Autodesk Inventor part; units mm, degrees
ref_plane "Work Plane6" through (0, -38.4796, -26.2038) normal (0, 0, -1) x (-1, 0, 0)
ref_plane "Work Plane3" through (0, 0, 0) normal (-1, 0, 0) x (0, 0, 1)
ref_plane "Work Plane1" through (0, -38.4796, -36.2038) normal (0, 0, -1) x (-1, 0, 0)
sketch "Sketch1" plane through (0, 0, 0) normal (1, 0, 0) x (0, 1, 0)
  circle A0 centre (-12.8712, -19.8017) radius 2.1703
  circle A1 centre (-32.0775, -0.5955) radius 2.1703
  circle A2 centre (31.9433, -0.5955) radius 2.1703
  circle A3 centre (31.9433, 13.4891) radius 2.1703
  circle A4 centre (-32.0775, 13.4891) radius 2.1703
  circle A5 centre (12.7371, -19.8017) radius 2.1703
  line L0 (38.3454, 26.2933) -> (38.3454, -26.2038)
  line L1 (-38.4796, 26.2933) -> (38.3454, 26.2933)
  line L2 (-38.4796, 26.2933) -> (-38.4796, -26.2038)
  line L3 (38.3454, -26.2038) -> (-38.4796, -26.2038)
  circle A6 centre (-32.0775, 13.4891) radius 2.1703
  circle A7 centre (-32.0775, -0.5955) radius 2.1703
  line L4 (11.5, -7) -> (-11.5, -7)
  line L5 (-11.5, -7) -> (-11.5, 7)
  line L6 (-11.5, 7) -> (11.5, 7)
  line L7 (11.5, 7) -> (11.5, -7)
  line L8 (11.5, -7) -> (-11.5, 7) construction
  line L9 (-11.5, -7) -> (11.5, 7) construction
  circle A8 centre (13.2, 0) radius 1
  circle A9 centre (-14, 0) radius 1
  point P0 (0, 0)
  point P1 (-11.5, 0)
  dimension "d26" = 23
  dimension "d27" = 14
  dimension "d28" = 27.2
  dimension "d29" = 2
  dimension "d30" = 2.5
ref_plane "Work Plane6" through (0, -38.4796, -26.2038) normal (0, 0, -1) x (-1, 0, 0)
sketch "Sketch3" plane through (0, -38.4796, -26.2038) normal (0, 0, -1) x (-1, 0, 0)
  line L0 (0, 76.825) -> (-3, 76.825)
  line L1 (0, 0) -> (-3, 0)
  line L2 (-3, 76.825) -> (0, 76.825)
  line L3 (0, 76.825) -> (0, 0)
  line L4 (0, 0) -> (-3, 0)
  line L5 (-3, 0) -> (-3, 76.825)
  line L6 (0, 0) -> (0, 76.825)
  line L7 (-3, 0) -> (-3, 76.825)
  line L8 (0.01, -0.01) -> (0.01, 76.835)
  line L9 (0.01, 76.835) -> (-3.01, 76.835)
  line L10 (-3.01, 76.835) -> (-3.01, -0.01)
  line L11 (-3.01, -0.01) -> (0.01, -0.01)
  point P0 (0, 38.4796)
  dimension "d3" = 0.01
extrude "Extrusion2" add sketch "Sketch3" along normal blind 10 contours L3 L1 L5 L0
ref_plane "Work Plane3" through (0, 0, 0) normal (-1, 0, 0) x (0, 0, 1)
sketch "Sketch4" plane through (0, 0, 0) normal (-1, 0, 0) x (0, 0, 1)
  line L0 (26.2933, -38.4796) -> (-36.2038, -38.4796)
  line L1 (-36.2038, 38.422) -> (-33.2038, 38.422)
  line L2 (-33.2038, 38.422) -> (-33.2038, -38.4796)
  line L3 (-33.2038, -38.4796) -> (-36.2038, -38.4796)
  line L4 (-36.2038, -38.4796) -> (-36.2038, 38.422)
  line L5 (-36.2038, 38.3454) -> (-36.2038, -38.4796)
  point P0 (0, 0)
  dimension "d8" = 3
extrude "Extrusion3" add sketch "Sketch4" against normal blind 60
ref_plane "Work Plane1" through (0, -38.4796, -36.2038) normal (0, 0, -1) x (-1, 0, 0)
ref_plane "Work Plane4" through (0, -38.4796, -36.2038) normal (0, 0, -1) x (-1, 0, 0)
sketch "Sketch6" plane through (0, -38.4796, -36.2038) normal (0, 0, -1) x (-1, 0, 0)
  line L0 (0, 38.4796) -> (-60, 38.4508)
  line L1 (-60, 0) -> (-60, 76.9016)
  line L2 (-30, 76.2766) -> (-30, 0)
  line L3 (-43.0944, 47.6588) -> (-43.0944, 27.6588)
  arc A0 (-47.5944, 27.6588) -> (-43.0944, 27.6588) centre (-45.3444, 27.6588) ccw
  line L4 (-47.5944, 27.6588) -> (-47.5944, 47.6588)
  arc A1 (-43.0944, 47.6588) -> (-47.5944, 47.6588) centre (-45.3444, 47.6588) ccw
  circle A2 centre (-35, 27.8243) radius 1
  circle A3 centre (-10, 27.8243) radius 1
  circle A4 centre (-35, 48.8243) radius 1
  circle A5 centre (-10, 48.8243) radius 1
  line L5 (-57.8444, 58.6588) -> (-57.8444, 17.5214)
  line L6 (-57.8444, 17.5214) -> (-2.3444, 17.5214)
  line L7 (-2.3444, 17.5214) -> (-2.3444, 58.6588)
  line L8 (-2.3444, 58.6588) -> (-57.8444, 58.6588)
  line L9 (-57.8444, 58.6588) -> (-60, 58.6588)
  line L10 (-2.3444, 58.6588) -> (0, 58.6588)
  line L11 (0, 58.6588) -> (0, 17.5214)
  line L12 (0, 17.5214) -> (-2.3444, 17.5214)
  line L13 (-57.8444, 17.5214) -> (-60, 17.5214)
  line L14 (0, 0) -> (-60, 0)
  line L15 (-7.6908, 17.5214) -> (-60, 17.5214)
  line L16 (-60, 17.5214) -> (-60, 0)
  line L17 (-60, 0) -> (-7.6908, 0)
  line L18 (-7.6908, 0) -> (-7.6908, 17.5214)
  line L19 (-7.6908, 76.2766) -> (-60, 76.2766)
  line L20 (-60, 76.2766) -> (-60, 58.6588)
  line L21 (-60, 58.6588) -> (-7.6908, 58.6588)
  line L22 (-7.6908, 58.6588) -> (-7.6908, 76.2766)
  point P0 (0, 76.9016)
  point P1 (-57.8444, 34.2959)
  dimension "d12" = 25
  dimension "d13" = 35
  dimension "d14" = 35
  dimension "d15" = 25
extrude "Extrusion4" cut sketch "Sketch6" against normal blind 60 contours L3 A0 L4 L0 | L0 L4 A1 L3 | L8 L9 L1 L19 L2 | L2 L19 L22 L8 | L6 L18 L14 L2 | L2 L14 L1 L13 L6 | A2 | A3 | A4 | A5
sketch "Sketch7" plane through (0, -38.4796, -36.2038) normal (0, 0, -1) x (-1, 0, 0)
  point P0 (0, 38.4796)
extrude "Extrusion7" add sketch "Sketch1" against normal blind 2
ref_plane "Work Plane7" through (0, 38.422, -36.2038) normal (-1, 0, 0) x (0, 0, 1)
sketch "Sketch9" plane through (0, 38.422, -36.2038) normal (-1, 0, 0) x (0, 0, 1)
  line L0 (0, -76.9016) -> (0, 0)
  line L1 (0, 0) -> (10, 0)
  line L2 (10, 0) -> (10, -76.9016)
  line L3 (10, -76.9016) -> (0, -76.9016)
  line L4 (0, -76.9016) -> (0, 0)
  point P0 (36.2038, -38.422)
extrude "Extrusion8" add sketch "Sketch9" along normal blind 2
sketch "Sketch10" plane through (60, 0, 0) normal (1, 0, 0) x (0, 0, -1)
  line L0 (36.2038, 38.422) -> (33.2038, 38.422)
  line L1 (33.2038, 37.797) -> (36.2038, 37.797)
  line L2 (33.2038, 38.422) -> (36.2038, 38.422)
  line L3 (36.2038, 38.422) -> (36.2038, 37.797)
  line L4 (36.2038, 37.797) -> (33.2038, 37.797)
  line L5 (33.2038, 37.797) -> (33.2038, 38.422)
  point P0 (0, 0)
extrude "Extrusion9" cut sketch "Sketch10" against normal blind 60.25
properties part number "cameramount"
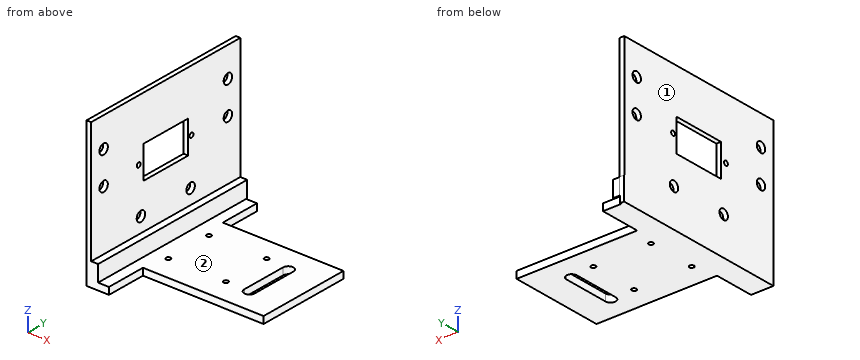
The model under review builds one solid part; all positions refer to its coordinate system, in mm. Face numbers are marked on the shaded views. A direction names the side the tool comes from. Coordinates: 2 decimals unless noted, no trailing zeros. Order: outer loops, then holes, each group sorted by start corner. A loop starts at its lowest first (then second) coordinate and runs counter-clockwise, first axis right, second up. Notation, with made-up numbers: (71.5, 51) -> (76.5, 51) arc R19 ccw to (76.5, 80) -> close; hole circle Ø4 at (-9.5, -26). An arc over 180 degrees is marked (long way). Answer in a Markdown table with one row per item.
(1) Wall thickness on line 1 along Y through (x, z) = (10, -35.4); line 2 along Z through (x, y) = (1, 18); line 3 along Z through (x, y) = (18.5, 6.5): over which ranges is each line inside the solid? List them lowest first.
Answers:
| item | result |
|---|---|
| line 1 | -20.96 to -11.66, -9.66 to 9.34, 11.34 to 20.18 |
| line 2 | -36.2 to -26.2 |
| line 3 | -36.2 to -33.2 |
(2) Consider section C-C (y = 13.2). Write out the cut boundary in (x, z), plus the area to 3 significant figures.
Answers:
| item | result |
|---|---|
| outline | (-2, -36.2) -> (60, -36.2) -> (60, -33.2) -> (3, -33.2) -> (3, -26.2) -> (0, -26.2) -> (0, -21.92) -> (-2, -21.92) -> close; (-2, -17.68) -> (0, -17.68) -> (0, -1) -> (-2, -1) -> close; (-2, 1) -> (0, 1) -> (0, 26.29) -> (-2, 26.29) -> close |
| area | 314 mm² |
(3) Consider section A-A (x = 10). Write out the cut boundary in (y, z).
Answers:
| item | result |
|---|---|
| outline | (-20.96, -36.2) -> (-11.66, -36.2) -> (-11.66, -33.2) -> (-20.96, -33.2) -> close; (-9.66, -36.2) -> (9.34, -36.2) -> (9.34, -33.2) -> (-9.66, -33.2) -> close; (11.34, -36.2) -> (20.18, -36.2) -> (20.18, -33.2) -> (11.34, -33.2) -> close |
(4) Consider section D-D (z = -24). Write out the cut boundary in (x, y), plus the area to 3 significant figures.
Answers:
| item | result |
|---|---|
| outline | (-2, -38.48) -> (0, -38.48) -> (0, 38.35) -> (-2, 38.35) -> close |
| area | 154 mm² |
(5) Consider section B-B (y = -20). Write out the cut boundary in (x, z).
Answers:
| item | result |
|---|---|
| outline | (-2, -36.2) -> (60, -36.2) -> (60, -33.2) -> (3, -33.2) -> (3, -26.2) -> (0, -26.2) -> (0, 26.29) -> (-2, 26.29) -> close |
(6) Insertion check: pin 1 (0.9 mm diameter, centred on x = 34.5, z = -35, fed in from +Y); pin 2 (2.5 mm diameter, centred on x = 10, y = 10.34, fed in from +Z); pin 3 (3.5 mm diameter, centred on y = 14.5, z = -31, fed in from +X). Each pin has a flat end and moves straight along its axis. Give the tip position at first contact, or say it passes through.
Answers:
| item | result |
|---|---|
| pin 1 | y = 20.18 |
| pin 2 | z = -33.2 |
| pin 3 | x = 3 |
(7) Machinability: for the marked faces 1 and 2, which of the approach directions +Z, -Z, +X, -X, +Y, -Y give a long, thin tool a straight path to every point of the face, cutting with its end or side? Answer none if there is none.
Answers:
| item | result |
|---|---|
| face 1 | +Z, -Z, -X, +Y, -Y |
| face 2 | +Z, +X, +Y, -Y |
